```python
from build123d import *

# Parameters (mm, degrees)
SKETCH1_R      = 2.35
SKETCH1_W      = 4
SKETCH1_H      = 3.1
EXTRUDE1_DEPTH = 3.1


with BuildPart() as part:
    # Sketch1 → Extrude1 (new body)
    with BuildSketch(Plane(origin=(0, 0, 0), x_dir=(1, 0, 0), z_dir=(0, 1, 0))):
        with BuildLine():
            Line((-41.013157114, 29.408489293), (-41.013157114, 26.058489293))
            ThreePointArc((-41.013157114, 26.058489293), (-40.689672648, 24.508533678), (-39.773228128, 23.217358224))
            Line((-39.773228128, 23.217358224), (-28.398228128, 12.667358224))
            ThreePointArc((-28.398228128, 12.667358224), (-25.763157114, 11.633489293), (-23.1280861, 12.667358224))
            Line((-23.1280861, 12.667358224), (-11.7530861, 23.217358224))
            ThreePointArc((-11.7530861, 23.217358224), (-10.83664158, 24.508533678), (-10.513157114, 26.058489293))
            Line((-10.513157114, 26.058489293), (-10.513157114, 29.408489293))
            Line((-10.513157114, 29.408489293), (-18.263157114, 29.408489293))
            Line((-18.263157114, 29.408489293), (-18.263157114, 32.508489293))
            Line((-18.263157114, 32.508489293), (-10.513157114, 32.508489293))
            Line((-10.513157114, 32.508489293), (-10.498924525, 34.508489293))
            Line((-10.498924525, 34.508489293), (-41.027382287, 34.508489293))
            Line((-41.027382287, 34.508489293), (-41.013157114, 32.508489293))
            Line((-41.013157114, 32.508489293), (-33.263157114, 32.508489293))
            Line((-33.263157114, 32.508489293), (-33.263157114, 29.408489293))
            Line((-33.263157114, 29.408489293), (-41.013157114, 29.408489293))
        make_face()
        with Locations(Location((-14.388157114, 26.058489293, 0), (0, 0, 90))):
            Circle(SKETCH1_R, mode=Mode.SUBTRACT)
        with Locations(Location((-37.138157114, 26.058489293, 0), (0, 0, 90))):
            Circle(SKETCH1_R, mode=Mode.SUBTRACT)
        with Locations(Location((-25.763157114, 15.508489293, 0), (0, 0, 90))):
            Circle(SKETCH1_R, mode=Mode.SUBTRACT)
        with BuildLine():
            Line((-33.76750302, 22.568552775), (-31.002944054, 20.130132194))
            Line((-31.002944054, 20.130132194), (-30.638157114, 20.130132194))
            ThreePointArc((-30.638157114, 20.130132194), (-29.931050333, 20.423025412), (-29.638157114, 21.130132194))
            Line((-29.638157114, 21.130132194), (-29.638157114, 22.458489293))
            ThreePointArc((-29.638157114, 22.458489293), (-29.345263895, 23.165596075), (-28.638157114, 23.458489293))
            Line((-28.638157114, 23.458489293), (-22.889213944, 23.458489293))
            ThreePointArc((-22.889213944, 23.458489293), (-22.182388419, 23.165877219), (-21.889214261, 22.459284647))
            Line((-21.889214261, 22.459284647), (-21.888157114, 21.130132194))
            ThreePointArc((-21.888157114, 21.130132194), (-21.595263895, 20.423025412), (-20.888157114, 20.130132194))
            Line((-20.888157114, 20.130132194), (-20.523370174, 20.130132194))
            Line((-20.523370174, 20.130132194), (-17.758811208, 22.568552775))
            ThreePointArc((-17.758811208, 22.568552775), (-17.428169762, 23.19327051), (-17.593190704, 23.880558008))
            ThreePointArc((-17.593190704, 23.880558008), (-17.720651816, 24.081090988), (-17.835582513, 24.289059126))
            ThreePointArc((-17.835582513, 24.289059126), (-18.600140603, 25.542598068), (-19.540017718, 26.670667198))
            Line((-19.540017718, 26.670667198), (-21.890008982, 29.103277241))
            ThreePointArc((-21.890008982, 29.103277241), (-22.218575416, 29.329029338), (-22.609223629, 29.408489293))
            Line((-22.609223629, 29.408489293), (-28.917090599, 29.408489293))
            ThreePointArc((-28.917090599, 29.408489293), (-29.307738812, 29.329029338), (-29.636305246, 29.103277241))
            Line((-29.636305246, 29.103277241), (-31.98629651, 26.670667198))
            ThreePointArc((-31.98629651, 26.670667198), (-32.926173625, 25.542598068), (-33.690731715, 24.289059126))
            ThreePointArc((-33.690731715, 24.289059126), (-33.805662411, 24.081090988), (-33.933123524, 23.880558008))
            ThreePointArc((-33.933123524, 23.880558008), (-34.098144466, 23.19327051), (-33.76750302, 22.568552775))
        make_face(mode=Mode.SUBTRACT)
        with Locations((-25.763157114, 20.408489293)):
            Rectangle(SKETCH1_W, SKETCH1_H, mode=Mode.SUBTRACT)
    extrude(amount=EXTRUDE1_DEPTH)


solid = part.part
```
Here's how the part is built. I have some questions about the finished solid (model axes, mm). A direction names the side the tool comes from. Coordinates: 2 decimals unless noted, no trailing zeros. Write each loop counter-clockwise with the first axis right and the second up, starting at its lowest first coordinate (ties: lowest second). Pieces come first, ordered by that corner, then holes. Notation, with made-up numbers: (39, 74) -> (61, 74) arc R24 cw to (61, 97) -> close; hole circle Ø6 at (66.5, -11). An arc over 180 degrees is marked (long way). Use a Markdown table: item, result. Add a question column.
(1) We'd pull the mould along Z, two halves only. Please class faces 1 (the flat face through (-26, 2, -34.508)), 2 (the cylindrical face through (-13.49, 1.53, -28.23)), 3 (the cylindrical face through (-40.7, 1.53, -24.53)), 4 (the flat face through (-26, 0, -23)): +Z half, -Z half, draft (parallel to the pull), parting line (faces both ways), or undercut.
(2) If we section it at B-B, the plane x = -16: Write out the boundary of the cut face in (y, z), and give its area (3 significant figures).
(3) For faces 5 (the flat face through (-18.263, 2, -31)), 6 (the flat face through (-26, 2, -21.958)), which set-ups out of +Z, -Z, +X, -X, +Y, -Y let a thin tool reach every point of the face, with its end or its side?
(4) If we section it at D-D, the plane y = 0.95: State how many separate pieces and enclosed holes the cut face has, and give its area (3 significant figures).
(5) Please list where these lines run through material, in increasing order: line 1 (X direction, y = 2.1, z = -27.25); line 2 (Z direction, x = -27, y = 0.9); line 3 (Z direction, x = -25, y = 0.35).
(6) If we section it at C-C, the plane z = -31: Write out the boundary of the cut face in (x, y), and give its area (3 significant figures).
(7) I'm going to push flat-ended pins straight in: P1, Ø1.6, axis at x = -14.5, y = 2, coming from the +Z side; P2, Ø8, axis at x = -27, z = -15, coming from the -Y side; P3, Ø1, axis at x = -18, y = 0.5, coming from the +Z side; P4, Ø1.6, axis at y = 1.5, z = -27.5, coming from the +X side. Where does each tip first touch, or does it pass through?
(8) If we section it at A-A, the plane x = -27: Write out the boundary of the cut face in (y, z), and give its area (3 significant figures).
Outcome:
| question | item | result |
|---|---|---|
| 1 | face 1 | -Z half |
| 1 | face 2 | undercut |
| 1 | face 3 | +Z half |
| 1 | face 4 | draft |
| 2 | outline | (0, -34.51) -> (3.1, -34.51) -> (3.1, -32.51) -> (0, -32.51) -> close; (0, -29.41) -> (3.1, -29.41) -> (3.1, -27.77) -> (0, -27.77) -> close; (0, -24.35) -> (3.1, -24.35) -> (3.1, -19.28) -> (0, -19.28) -> close |
| 2 | area | 27.0 mm^2 |
| 3 | face 5 | +X, +Y, -Y |
| 3 | face 6 | +Y, -Y |
| 4 | separate pieces | 1 |
| 4 | enclosed holes | 5 |
| 4 | area | 313 mm^2 |
| 5 | line 1 | x = -41.01 to -39.16, -35.11 to -31.43, -20.1 to -16.41, -12.36 to -10.51 |
| 5 | line 2 | z = -34.51 to -29.41, -23.46 to -21.96, -18.86 to -17.51, -13.51 to -11.84 |
| 5 | line 3 | z = -34.51 to -29.41, -23.46 to -21.96, -18.86 to -17.73, -13.29 to -11.71 |
| 6 | outline | (-33.26, 0) -> (-18.26, 0) -> (-18.26, 3.1) -> (-33.26, 3.1) -> close |
| 6 | area | 46.5 mm^2 |
| 7 | P1 | stops at z = -19.93 |
| 7 | P2 | stops at y = 0 |
| 7 | P3 | stops at z = -16.96 |
| 7 | P4 | stops at x = -10.51 |
| 8 | outline | (0, -34.51) -> (3.1, -34.51) -> (3.1, -29.41) -> (0, -29.41) -> close; (0, -23.46) -> (3.1, -23.46) -> (3.1, -21.96) -> (0, -21.96) -> close; (0, -18.86) -> (3.1, -18.86) -> (3.1, -17.51) -> (0, -17.51) -> close; (0, -13.51) -> (3.1, -13.51) -> (3.1, -11.84) -> (0, -11.84) -> close |
| 8 | area | 29.8 mm^2 |
